```python
from build123d import *

# Parameters (mm, degrees)
F0_W     = 44.45
F0_H     = 4.7625
F1_DEPTH = 38.1
F3_D     = 6.35
F4_R     = 5.08


with BuildPart() as f1:
    # F0 (on Front) → F1 (new body)
    with BuildSketch(Plane.XZ):
        Polygon((-22.225, -2.38125), (-22.225, 2.38125), (-22.225, 10.31875), (-38.1, 10.31875), (-38.1, -2.38125), align=None)
        Rectangle(F0_W, F0_H)
        Polygon((22.225, 10.31875), (22.225, 2.38125), (22.225, -2.38125), (38.1, -2.38125), (38.1, 10.31875), align=None)
    extrude(amount=F1_DEPTH)

    # F3 (through all)
    with Locations(Plane.XY.offset(10.31875)):
        with Locations((-30.1625, -9.525), (-30.1625, -28.575), (30.1625, -9.525), (30.1625, -28.575)):
            Hole(F3_D / 2)

    # F4
    f4_edges = [f1.edges().sort_by_distance(p)[0] for p in [
        (38.1, 0, 3.96875),
        (38.1, -38.1, 3.96875),
        (-38.1, 0, 3.96875),
        (-38.1, -38.1, 3.96875),
    ]]
    fillet(f4_edges, radius=F4_R)


solid = f1.part
```
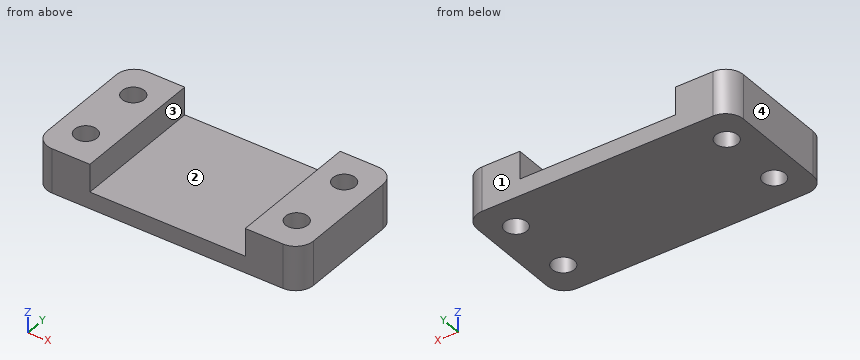
Check sheet for the modelled part. Datum: model origin and axes. Units: mm. Face numbers are marked on the shaded views. Give positions to 0.01 mm unless a question says otherwise; leave off trailing zeros. Order: outer loops, then holes, each group sorted by start corner. A loop starts at its lowest first (then second) coordinate and runs counter-clockwise, first axis right, second up. Notation, with made-up numbers: (-18.75, -15.75) -> (-10.75, -15.75) arc R26 ccw to (-10.75, 19.25) -> close; hole circle Ø7 at (3, 47.25). An arc over 180 degrees is marked (long way). Use CSV: the item, a comma, the result in double quotes. Start each with the question number.
1) Material ranges on line 1 (X direction, y = -12, z = 6) (3 decimals); line 2 (X direction, y = -33, z = 7) (3 decimals); line 3 (X direction, y = -31, z = 0.75), recorded low to high. Write a range as from..to.
2) Sectioned sample at D-D, the plane y = -14. Record the boundary of the cut face in (x, z) (3 decimals).
3) Sectioned sample at A-A, the plane z = 7.25. Give the number of separate pieces and of enclosed holes in the cut face, plus the area to 3 significant figures.
4) Sectioned sample at B-B, the plane y = -29.5. Record the boundary of the cut face in (x, z) (3 decimals), plus the area to 3 significant figures.
5) Go/stop test with flat-tipped pins: P1, Ø4, axis at x = -30.16, y = -28.58, coming from the -Z side; P2, Ø19, axis at x = 1, y = -24.5, coming from the +Z side. Record where each tip stops, or that it passes through.
6) Mould release check, pull along X, two halves, no side actions. Record for the marked faces 1, 2, 3 and 4: released by +X, released by -X, zero draft, split by the parting line, or undercut.
7) Sectioned sample at C-C, the plane x = -31. Record the boundary of the cut face in (y, z).
Recorded:
1,line 1,"-38.1..-32.151, -28.174..-22.225, 22.225..28.174, 32.151..38.1"
1,line 2,"-38.1..-22.225, 22.225..38.1"
1,line 3,"-38.1..-32.21, -28.11..28.11, 32.21..38.1"
2,outline,"(-38.1, -2.381) -> (38.1, -2.381) -> (38.1, 10.319) -> (22.225, 10.319) -> (22.225, 2.381) -> (-22.225, 2.381) -> (-22.225, 10.319) -> (-38.1, 10.319) -> close"
3,separate pieces,"2"
3,enclosed holes,"4"
3,area,"1,060 mm2"
4,outline,"(-38.1, -2.381) -> (-33.2, -2.381) -> (-33.2, 10.319) -> (-38.1, 10.319) -> close; (-27.125, -2.381) -> (27.125, -2.381) -> (27.125, 10.319) -> (22.225, 10.319) -> (22.225, 2.381) -> (-22.225, 2.381) -> (-22.225, 10.319) -> (-27.125, 10.319) -> close; (33.2, -2.381) -> (38.1, -2.381) -> (38.1, 10.319) -> (33.2, 10.319) -> close"
4,area,"461 mm2"
5,P1,"through"
5,P2,"z = 2.38"
6,face 1,"zero draft"
6,face 2,"undercut"
6,face 3,"undercut"
6,face 4,"released by -X"
7,outline,"(-38.1, -2.38) -> (-31.64, -2.38) -> (-31.64, 10.32) -> (-38.1, 10.32) -> close; (-25.51, -2.38) -> (-12.59, -2.38) -> (-12.59, 10.32) -> (-25.51, 10.32) -> close; (-6.46, -2.38) -> (0, -2.38) -> (0, 10.32) -> (-6.46, 10.32) -> close"
